Geometry check sheet. Reference: the model listing, model coordinates, mm. Face numbers are marked on the shaded views. A direction names the side the tool comes from. Round coordinates to 2 decimals unless told otherwise and drop trailing zeros. Write each loop counter-clockwise with the first axis right and the second up, starting at its lowest first coordinate (ties: lowest second). Pieces come first, ordered by that corner, then holes. Notation, with made-up numbers: (-17, 78) - (12, 78) arc R26 ccw to (12, 93) - close; hole circle Ø4 at (10, 4). An arc over 180 degrees is marked (long way). Return JSON: item names as keys, results as strings.
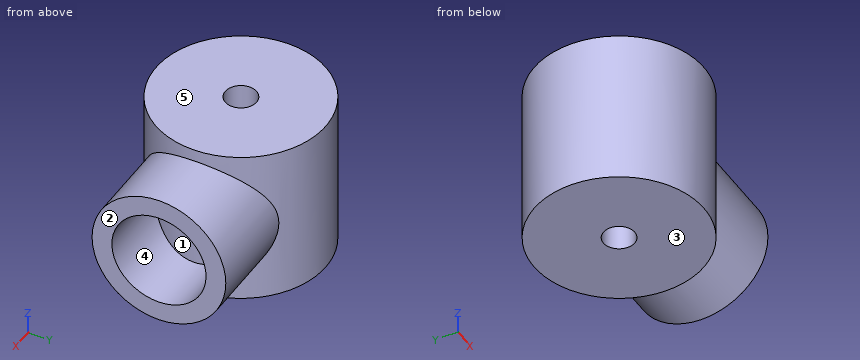
```python
from build123d import *

# Parameters (mm, degrees)
BOSS_EXTRUDE2_DEPTH      = 8
BOSS_EXTRUDE2_DEPTH_BACK = 8
SKETCH1_R                = 8.5875
SKETCH1_R_2              = 1.5875
SKETCH2_R                = 6.7625
SKETCH2_R_2              = 4.7625
BOSS_EXTRUDE3_DEPTH      = 15
CUT_EXTRUDE1_DEPTH       = 10
CUT_EXTRUDE1_DEPTH_BACK  = 10
SKETCH3_R                = 1.5875


with BuildPart() as part:
    # Sketch1 → Boss-Extrude2 (new, two sides: drawn at the far end of the back side and taken through both)
    with BuildSketch(Plane.XY.offset(-BOSS_EXTRUDE2_DEPTH_BACK)):
        Circle(SKETCH1_R)
        Circle(SKETCH1_R_2, mode=Mode.SUBTRACT)
    extrude(amount=BOSS_EXTRUDE2_DEPTH + BOSS_EXTRUDE2_DEPTH_BACK)

    # Sketch2 → Boss-Extrude3 (add)
    with BuildSketch(Plane(origin=(0, 0, 0), x_dir=(0, 0, -1), z_dir=(1, 0, 0))):
        Circle(SKETCH2_R)
        Circle(SKETCH2_R_2, mode=Mode.SUBTRACT)
    extrude(amount=BOSS_EXTRUDE3_DEPTH)

    # Sketch3 → Cut-Extrude1 (cut, two sides: drawn at the far end of the back side and taken through both)
    with BuildSketch(Plane.XY.offset(-CUT_EXTRUDE1_DEPTH_BACK)):
        Circle(SKETCH3_R)
    extrude(amount=CUT_EXTRUDE1_DEPTH + CUT_EXTRUDE1_DEPTH_BACK, mode=Mode.SUBTRACT)


solid = part.part
```
(1) Release check for a two-part mould opening along Z. For the marked faces 1, 2 and 3 record: pulls with the +Z half, pulls with the -Z half, needs draft (parallel to the pull), parting line crosses it, or undercut.
Response values:
{"face 1": "undercut", "face 2": "needs draft", "face 3": "pulls with the -Z half"}
(2) Access from +Z, -Z, +X, -X, +Y, -Y to the whole of each face (thin tool, end or side, straight path). Record for the marked faces 4 and 5.
Response values:
{"face 4": "+X", "face 5": "+Z, +X, -X, +Y, -Y"}
(3) Section check D-D, the plane y = 2.5. Enter the section's corners in (x, z).
Response values:
{"outline": "(-8.22, -8) - (8.22, -8) - (8.22, -6.28) - (15, -6.28) - (15, -4.05) - (8.22, -4.05) - (8.22, 4.05) - (15, 4.05) - (15, 6.28) - (8.22, 6.28) - (8.22, 8) - (-8.22, 8) - close"}
(4) Section check B-B, the plane x = 0. Enter the section's corners in (y, z), plus the area to 3 significant figures.
Response values:
{"outline": "(-8.59, -8) - (-1.59, -8) - (-1.59, 8) - (-8.59, 8) - close; (1.59, -8) - (8.59, -8) - (8.59, 8) - (1.59, 8) - close", "area": "224 mm^2"}
(5) Gauge pin test, flat ends, axial feed: pin 1 (3 mm diameter, centred on x = 7, z = 0, fed in from -Y); pin 2 (4 mm diameter, centred on y = -1, z = -0.5, fed in from +X); pin 3 (2 mm diameter, centred on y = -6.5, z = 4, fed in from -X). Record the tip position at first contact, or that the pin passes through.
Response values:
{"pin 1": "stops at y = -6.76", "pin 2": "stops at x = 8.59", "pin 3": "stops at x = -6.6"}
(6) Section check A-A, the plane y = 0. Enter the section's corners in (x, z).
Response values:
{"outline": "(-8.59, -8) - (-1.59, -8) - (-1.59, 8) - (-8.59, 8) - close; (1.59, -8) - (8.59, -8) - (8.59, -6.76) - (15, -6.76) - (15, -4.76) - (8.59, -4.76) - (8.59, 4.76) - (15, 4.76) - (15, 6.76) - (8.59, 6.76) - (8.59, 8) - (1.59, 8) - close"}
(7) Section check C-C, the plane z = 0. Enter the section's corners in (x, y) (1 decimal).
Response values:
{"outline": "(5.3, -6.8) - (15, -6.8) - (15, -4.8) - (7.1, -4.8) arc R8.6 ccw to (7.1, 4.8) - (15, 4.8) - (15, 6.8) - (5.3, 6.8) arc R8.6 ccw (long way) to start; hole circle Ø3.2 at (0, 0)"}
(8) Material ranges on line 1 along Z through (x, y) = (10.25, 0); line 2 along Y through (x, z) = (0, -0.75); line 3 along X through (y, z) = (0.5, 2.75), recorded low to high. Write a range as [from, to].
Response values:
{"line 1": "z = [-6.76, -4.76], [4.76, 6.76]", "line 2": "y = [-8.59, -1.59], [1.59, 8.59]", "line 3": "x = [-8.57, -1.51], [1.51, 8.57]"}
